```python
from build123d import *

# Parameters (mm, degrees)
MODEL_R             = 1.45
MODEL_R_2           = 1
BOSS_EXTRUDE1_DEPTH = 5.85


with BuildPart() as part:
    # Model → Boss-Extrude1 (new body)
    with BuildSketch(Plane.XY):
        with BuildLine():
            Line((508.182236888, 554.934833401), (506.087301785, 543.461595882))
            ThreePointArc((506.087301785, 543.461595882), (506.893587564, 539.980874482), (509.982236888, 538.184833401))
            Line((509.982236888, 538.184833401), (529.982236888, 538.184833401))
            ThreePointArc((529.982236888, 538.184833401), (533.070886212, 539.980874482), (533.877171991, 543.461595882))
            Line((533.877171991, 543.461595882), (531.782236888, 554.934833401))
            Line((531.782236888, 554.934833401), (531.782236888, 577.734833401))
            ThreePointArc((531.782236888, 577.734833401), (530.317770794, 581.270367307), (526.782236888, 582.734833401))
            Line((526.782236888, 582.734833401), (524.282236888, 582.734833401))
            Line((524.282236888, 582.734833401), (524.282236888, 576.984833401))
            Line((524.282236888, 576.984833401), (526.082236888, 576.984833401))
            Line((526.082236888, 576.984833401), (526.082236888, 554.184833401))
            Line((526.082236888, 554.184833401), (513.882236888, 554.184833401))
            Line((513.882236888, 554.184833401), (513.882236888, 576.984833401))
            Line((513.882236888, 576.984833401), (515.682236888, 576.984833401))
            Line((515.682236888, 576.984833401), (515.682236888, 582.734833401))
            Line((515.682236888, 582.734833401), (513.182236888, 582.734833401))
            ThreePointArc((513.182236888, 582.734833401), (509.646702982, 581.270367307), (508.182236888, 577.734833401))
            Line((508.182236888, 577.734833401), (508.182236888, 554.934833401))
        make_face()
        with Locations(Location((509.982236888, 542.184833401, 0), (0, 0, 180))):
            Circle(MODEL_R, mode=Mode.SUBTRACT)
        with Locations((519.982236888, 542.184833401)):
            Circle(MODEL_R, mode=Mode.SUBTRACT)
        with Locations((529.982236888, 542.184833401)):
            Circle(MODEL_R, mode=Mode.SUBTRACT)
        with Locations((519.982236888, 551.984833401)):
            Circle(MODEL_R_2, mode=Mode.SUBTRACT)
    extrude(amount=BOSS_EXTRUDE1_DEPTH)


solid = part.part
```
Check sheet for the modelled part. Datum: model origin and axes. Units: mm. A direction names the side the tool comes from. Coordinates: 2 decimals unless noted, no trailing zeros. Write each loop counter-clockwise with the first axis right and the second up, starting at its lowest first coordinate (ties: lowest second). Pieces come first, ordered by that corner, then holes. Notation, with made-up numbers: (52.5, 35) -> (99.5, 35) arc R35 cw to (99.5, 70) -> close; hole circle Ø8 at (15, 60.5). An arc over 180 degrees is marked (long way). Use a Markdown table: item, result.
1. Tool access check on faces 4 (the flat face through (515.682, 580, 3)), 5 (the flat face through (526.082, 566, 3)), 6 (the flat face through (508.182, 566, 3)). Record the directions out of +Z, -Z, +X, -X, +Y, -Y that give a thin tool (end or side, any length) a straight path to the whole face; none if there is none.
Reported:
| item | result |
|---|---|
| face 4 | +Z, -Z, +Y |
| face 5 | +Z, -Z |
| face 6 | +Z, -Z, -X, +Y |
2. Sectioned sample at C-C (z = 5.2). Enter the section's corners in (x, y).
Reported:
| item | result |
|---|---|
| outline | (506.09, 543.46) arc R4.5 ccw to (509.98, 538.18) -> (529.98, 538.18) arc R4.5 ccw to (533.88, 543.46) -> (531.78, 554.93) -> (531.78, 577.73) arc R5 ccw to (526.78, 582.73) -> (524.28, 582.73) -> (524.28, 576.98) -> (526.08, 576.98) -> (526.08, 554.18) -> (513.88, 554.18) -> (513.88, 576.98) -> (515.68, 576.98) -> (515.68, 582.73) -> (513.18, 582.73) arc R5 ccw to (508.18, 577.73) -> (508.18, 554.93) -> close; hole circle Ø2.9 at (509.98, 542.18); hole circle Ø2.9 at (519.98, 542.18); hole circle Ø2 at (519.98, 551.98); hole circle Ø2.9 at (529.98, 542.18) |
3. Sectioned sample at D-D (y = 545.5). Enter the section's corners in (x, z), plus the area to 3 significant figures.
Reported:
| item | result |
|---|---|
| outline | (506.46, 0) -> (533.5, 0) -> (533.5, 5.85) -> (506.46, 5.85) -> close |
| area | 158 mm2 |
4. Sectioned sample at A-A (x = 525). Enter the section's corners in (y, z).
Reported:
| item | result |
|---|---|
| outline | (538.18, 0) -> (554.18, 0) -> (554.18, 5.85) -> (538.18, 5.85) -> close; (576.98, 0) -> (582.73, 0) -> (582.73, 5.85) -> (576.98, 5.85) -> close |
5. Sectioned sample at B-B (y = 566.5). Enter the section's corners in (x, z).
Reported:
| item | result |
|---|---|
| outline | (508.18, 0) -> (513.88, 0) -> (513.88, 5.85) -> (508.18, 5.85) -> close; (526.08, 0) -> (531.78, 0) -> (531.78, 5.85) -> (526.08, 5.85) -> close |
6. Release check for a two-part mould opening along Y. For faces 1 (the flat face through (514, 582.735, 3)), 2 (the flat face through (513.6, 555.8, 0)), 3 (the flat face through (515, 576.985, 3)) record: pulls with the +Y half, pulls with the -Y half, needs draft (parallel to the pull), parting line crosses it, or undercut.
Reported:
| item | result |
|---|---|
| face 1 | pulls with the +Y half |
| face 2 | needs draft |
| face 3 | undercut |
7. Go/stop test with flat-tipped pins: pin 1 Ø1.8 at (y, z) = (560, 4) entering from +X; pin 2 Ø1.7 at (y, z) = (580, 3.5) entering from -X; pin 3 Ø3 at (y, z) = (560.5, 1.5) entering from -X. Record where each tip stops, or that it passes through.
Reported:
| item | result |
|---|---|
| pin 1 | stops at x = 531.78 |
| pin 2 | stops at x = 508.39 |
| pin 3 | stops at x = 508.18 |
8. Scan lines: line 1 along X through (y, z) = (567, 5.15); line 2 along Y through (x, z) = (514, 3.55); line 3 along Y through (x, z) = (509.75, 2.65). Record each from-to range of solid material in increasing order.
Reported:
| item | result |
|---|---|
| line 1 | x = 508.18 to 513.88, 526.08 to 531.78 |
| line 2 | y = 538.18 to 554.18, 576.98 to 582.73 |
| line 3 | y = 538.22 to 540.75, 543.62 to 581.37 |
